from build123d import *

# Parameters (mm, degrees)
SKETCH1_W           = 25.4
SKETCH1_H           = 1.5875
BOSS_EXTRUDE1_DEPTH = 5.588


with BuildPart() as part:
    # Sketch1 → Boss-Extrude1 (new body)
    # profile 1 of 2: a face of its own
    with BuildSketch(Plane(origin=(-94.488, 0, 0), x_dir=(0, -1, 0), z_dir=(-1, 0, 0))):
        Polygon((136.525, -196.85), (111.125, -196.85), (111.125, -203.2), (85.725, -203.2), (85.725, -196.85), (60.325, -196.85), (60.325, -682.625), (85.725, -682.625), (85.725, -679.45), (111.125, -679.45), (111.125, -682.625), (136.525, -682.625), align=None)
        with Locations((98.425, -456.40625)):
            Rectangle(SKETCH1_W, SKETCH1_H, mode=Mode.SUBTRACT)
    # profile 2 of 2: a face of its own
    with BuildSketch(Plane(origin=(-94.488, 0, 0), x_dir=(0, -1, 0), z_dir=(-1, 0, 0))):
        with BuildLine():
            Line((149.225, -203.2), (136.525, -203.2))
            Line((136.525, -203.2), (136.525, -290.406498707))
            ThreePointArc((136.525, -290.406498707), (137.30121982, -286.034603668), (139.534994681, -282.197126202))
            Line((139.534994681, -282.197126202), (184.118202659, -229.57294303))
            ThreePointArc((184.118202659, -229.57294303), (185.23509009, -227.654204297), (185.6232, -225.468256778))
            Line((185.6232, -225.468256778), (185.6232, -203.2))
            Line((185.6232, -203.2), (168.275, -203.2))
            Line((168.275, -203.2), (168.275, -196.85))
            Line((168.275, -196.85), (149.225, -196.85))
            Line((149.225, -196.85), (149.225, -203.2))
        make_face()
    extrude(amount=-BOSS_EXTRUDE1_DEPTH)


solid = part.part
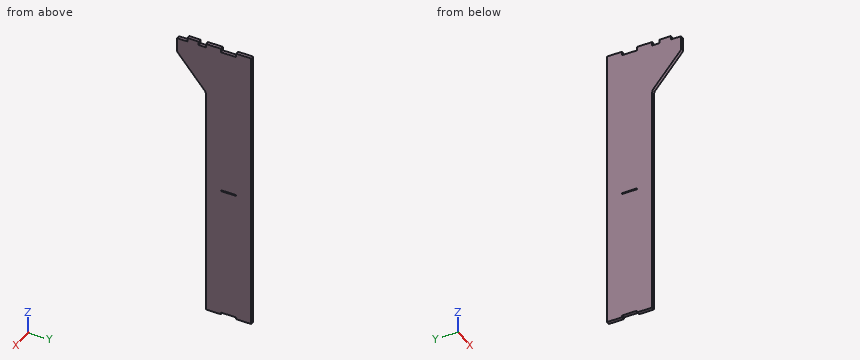
The listing builds one solid part. Answer for the finished solid, in the listing's coordinates (mm). Round coordinates to 2 decimals unless told otherwise and drop trailing zeros. Loops run counter-clockwise (first coordinate to the right, second up) from the corner with the lowest first, then second, coordinate; pieces in that order, holes last. Notation, with made-up numbers: M 61,81.25 L 94,81.25 A21 cw 94,116.25 Z; hole C 51,-39 d10. An arc over 180 degrees is marked long. Write each question's results on one line, items separated by ' | '. Start each with the question number.
1) Find section D-D on y = -174.5. Write down the section's boundary in (x, z), plus the area to 3 significant figures.
2) Straight lines are drawn through the part: probe 1 along Z at (x, y) = (-92.5, -108); probe 2 along Y at (x, z) = (-89.2, -503) (3 decimals); probe 3 along Z at (x, y) = (-94.05, -165.5). For each, find the intervals that lie inside material, in ascending order.
3) Find section A-A on y = -93. Write down the section's boundary in (x, z).
4) Find section C-C on z = -571.5. Write down the section's boundary in (x, y) (3 decimals).
5) Each of these flat-tipped pins is pushed along its axis until it touches: pin 1 (1.7 mm diameter, centred on x = -92.5, z = -498, fed in from -Y) (3 decimals); pin 2 (3 mm diameter, centred on x = -93, z = -198.5, fed in from -Y) (3 decimals); pin 3 (1.7 mm diameter, centred on x = -92, y = -102.5, fed in from -Z). Where does it stop, or does it pass through?
Final values:
1) outline: M -94.49,-240.93 L -88.9,-240.93 L -88.9,-203.2 L -94.49,-203.2 Z | area: 211 mm²
2) probe 1: -679.45 to -457.2, -455.61 to -203.2 | probe 2: -136.525 to -60.325 | probe 3: -251.55 to -196.85
3) outline: M -94.49,-679.45 L -88.9,-679.45 L -88.9,-457.2 L -94.49,-457.2 Z; M -94.49,-455.61 L -88.9,-455.61 L -88.9,-203.2 L -94.49,-203.2 Z
4) outline: M -94.488,-136.525 L -88.9,-136.525 L -88.9,-60.325 L -94.488,-60.325 Z
5) pin 1: y = -136.525 | pin 2: y = -168.275 | pin 3: z = -679.45
